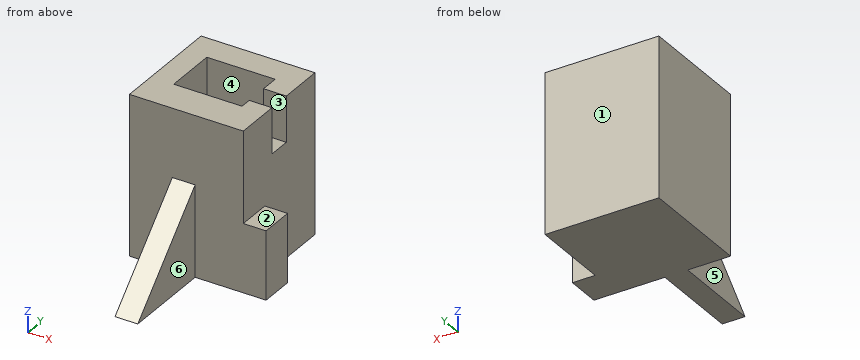
from build123d import *

# Parameters (mm, degrees)
F0_W      = 25
F0_H      = 25
F1_DEPTH  = 35
F2_W      = 7.5
F2_H      = 15
F3_DEPTH  = 5
F4_W      = 5
F4_H      = 5
F5_DEPTH  = 10
F7_DEPTH  = 18
F8_W      = 5
F8_H      = 20
F9_DEPTH  = 20
F11_DEPTH = 29.5


with BuildPart() as f1:
    # F0 (on Top) → F1 (new body)
    with BuildSketch(Plane.XY):
        with Locations((-0.820497, -3.517498)):
            Rectangle(F0_W, F0_H)
    extrude(amount=F1_DEPTH)

    # F2 (on face) → F3 (join)
    with BuildSketch(Plane.YZ.offset(11.679503)):
        with Locations((-12.267498, 7.5)):
            Rectangle(F2_W, F2_H)
    extrude(amount=F3_DEPTH)

    # F4 (on face) → F5 (cut)
    with BuildSketch(Plane.XY.offset(35)):
        with Locations((9.179503, -3.517498)):
            Rectangle(F4_W, F4_H)
    extrude(amount=-F5_DEPTH, mode=Mode.SUBTRACT)

    # F6 (on face) → F7 (cut)
    with BuildSketch(Plane.XY.offset(35)):
        Polygon((6.679503, 3.030628), (-8.320497, 3.030628), (-8.320497, -8.517498), (6.679503, -8.517498), (6.679503, -6.017498), (6.679503, -1.017498), align=None)
    extrude(amount=-F7_DEPTH, mode=Mode.SUBTRACT)

    # F8 (on face) → F9 (join)
    with BuildSketch(Plane.XZ.offset(16.017498)):
        with Locations((-1.402237, 10)):
            Rectangle(F8_W, F8_H)
    extrude(amount=F9_DEPTH)

    # F10 (on face) → F11 (cut)
    with BuildSketch(Plane(origin=(-3.902237, 0, 0), x_dir=(0, -1, 0), z_dir=(-1, 0, 0))):
        Polygon((36.017498, 20), (16.017498, 20), (36.017498, 0), align=None)
    extrude(amount=-F11_DEPTH, mode=Mode.SUBTRACT)


solid = f1.part
Work out the finished part from the listing and answer in its coordinate system (mm). Face numbers are marked on the shaded views. A direction names the side the tool comes from. Round coordinates to 2 decimals unless told otherwise and drop trailing zeros. Loops run counter-clockwise (first coordinate to the right, second up) from the corner with the lowest first, then second, coordinate; pieces in that order, holes last. Notation, with made-up numbers: (-27, 71.25) - (21, 71.25) arc R16 cw to (21, 96.25) - close; hole circle Ø1 at (86, 53). An arc over 180 degrees is marked (long way). Use one line per item in the form item = value. Start each with the question number.
(1) Determine the mould class of the marked faces 1, 2 and 3 for opening direction Y: +Y half, -Y half, draft (parallel to the pull), parting line (faces both ways), or undercut.
(2) Find section B-B on y = -2.5. Determine the outline of the cut face in (x, z), and give its area (3 significant figures).
(3) Consider line 1 (Y direction, x = 6, z = 29.5); line 2 (Z direction, x = 2, y = -2); line 3 (X direction, y = -7.5, z = 9). Determine where each line is inside the solid, lowest interval first.
(4) Find section C-C on x = 4.5. Determine the outline of the cut face in (y, z).
(5) Which of the six approach directions +Z, -Z, +X, -X, +Y, -Y give full straight-line access (tool end or side, diameter ignored) to the marked faces 4, 5 and 6?
(6) Find section D-D on z = 32. Determine the outline of the cut face in (x, y).
(7) Find section A-A on z = 24. Determine the outline of the cut face in (x, y).
(8) Flat-ended cylindrical pins translate along their axes: P1, Ø2, axis at y = -28, z = 4.5, coming from the -X side; P2, Ø12, axis at y = 2, z = 7, coming from the +X side; P3, Ø2.5, axis at x = 13.5, z = 4.5, coming from the +Y side; P4, Ø5.5, axis at x = 8.5, y = -4, coming from the +Z side. Find the tip coordinate at first contact, or state that the pin passes through.
Answer list:
q1.face_1 = +Y half
q1.face_2 = draft
q1.face_3 = undercut
q2.outline = (-13.32, 0) - (11.68, 0) - (11.68, 25) - (6.68, 25) - (6.68, 17) - (-8.32, 17) - (-8.32, 35) - (-13.32, 35) - close
q2.area = 555 mm^2
q3.line_1 = -16.02 to -8.52, 3.03 to 8.98
q3.line_2 = 0 to 17
q3.line_3 = -13.32 to 11.68
q4.outline = (-16.02, 0) - (8.98, 0) - (8.98, 35) - (3.03, 35) - (3.03, 17) - (-8.52, 17) - (-8.52, 35) - (-16.02, 35) - close
q5.face_4 = +Z
q5.face_5 = +Z, -Z, -X, -Y
q5.face_6 = +Z, -Z, +X, -Y
q6.outline = (-13.32, -16.02) - (11.68, -16.02) - (11.68, -6.02) - (6.68, -6.02) - (6.68, -8.52) - (-8.32, -8.52) - (-8.32, 3.03) - (6.68, 3.03) - (6.68, -1.02) - (11.68, -1.02) - (11.68, 8.98) - (-13.32, 8.98) - close
q7.outline = (-13.32, -16.02) - (11.68, -16.02) - (11.68, 8.98) - (-13.32, 8.98) - close; hole (-8.32, -8.52) - (6.68, -8.52) - (6.68, 3.03) - (-8.32, 3.03) - close
q8.P1 = -3.9
q8.P2 = 11.68
q8.P3 = -8.52
q8.P4 = 35
